Can you work these out from the model? Positions are in its coordinate system, mm. A direction names the side the tool comes from. Round coordinates to 2 decimals unless told otherwise and drop trailing zeros. Loops run counter-clockwise (first coordinate to the right, second up) from the corner with the lowest first, then second, coordinate; pieces in that order, holes last.
```python
from build123d import *

# Parameters (mm, degrees)
F1_DEPTH      = 6.4897
F1_DEPTH_BACK = 6.4897
F2_W          = 85.5599
F2_H          = 54.0004
F3_DEPTH      = 5.7277
F3_DEPTH_BACK = 5.7277
F4_R          = 0.762


with BuildPart() as f1:
    # F0 (on Top) → F1 (new body, two sides)
    with BuildSketch(Plane.XY) as f1_sk:
        Polygon((9.525, -27.7622), (9.525, 27.7622), (-9.525, 27.7622), (-9.525, 9.525), (-43.54195, 9.525), (-43.54195, -9.525), (-9.525, -9.525), (-9.525, -27.7622), align=None)
    extrude(amount=F1_DEPTH)
    extrude(f1_sk.sketch, amount=-F1_DEPTH_BACK)

    # F2 (on Top) → F3 (cut, two sides)
    with BuildSketch(Plane.XY) as f3_sk:
        Rectangle(F2_W, F2_H)
    extrude(amount=-F3_DEPTH, mode=Mode.SUBTRACT)
    extrude(f3_sk.sketch, amount=F3_DEPTH_BACK, mode=Mode.SUBTRACT)

    # F4
    f4_edges = [f1.edges().sort_by_distance(p)[0] for p in [
        (0, -27.7622, 6.4897),
        (0, -27.7622, -6.4897),
        (0, 27.7622, 6.4897),
        (0, 27.7622, -6.4897),
        (-43.54195, 0, -6.4897),
        (-43.54195, 0, 6.4897),
    ]]
    fillet(f4_edges, radius=F4_R)


solid = f1.part
```
(1) Which directions (+Z, -Z, +X, -X, +Y, -Y) give clear straight access to the entire face, cutting with the end or side of a thin tool? Please do faces 1 (the flat face through (-29, 9.525, -6)), 2 (the flat face through (-9.525, -20, -6)), 3 (the flat face through (0, 27, 0)), 4 (the flat face through (-11, 0, -5.728)), 5 (the flat face through (-42.78, 0, 0)).
(2) We'd pull the mould along Y, two halves only. Please class faces 6 (the flat face through (-9.525, 20, -6)), 7 (the flat face through (0, -27, 0)), 8 (the flat face through (0, -27.762, 0)): released by +Y, released by -Y, zero draft, split by the parting line, or undercut.
(3) Suppose I cut it at B-B (x = -18). Write out the boundary of the cut face in (y, z) (3 decimals), then the cut area to 3 significant figures.
(4) Suppose I cut it at D-D (x = 5.5). Write out the boundary of the cut face in (y, z).
(5) If I drill on line 1 (Z direction, x = -14.5, y = -3.5); line 2 (Y direction, x = 5, z = -3.5); line 3 (X direction, y = 2, z = -5.25), over which ranges is the centre line in solid material (lowest first)?
(6) Suppose I cut it at A-A (z = -2). Write out the boundary of the cut face in (x, y) (3 decimals).
Check result:
1. face 1: +Z, -Z, -X, +Y
1. face 2: +Z, -Z, -X, -Y
1. face 3: +X, -X
1. face 4: +X
1. face 5: +X, +Y, -Y
2. face 6: zero draft
2. face 7: undercut
2. face 8: released by -Y
3. outline: (-9.525, -6.49) - (9.525, -6.49) - (9.525, -5.728) - (-9.525, -5.728) - close; (-9.525, 5.728) - (9.525, 5.728) - (9.525, 6.49) - (-9.525, 6.49) - close
3. area: 29.0 mm2
4. outline: (-27.76, -5.73) arc R0.76 ccw to (-27, -6.49) - (27, -6.49) arc R0.76 ccw to (27.76, -5.73) - (27.76, 5.73) arc R0.76 ccw to (27, 6.49) - (-27, 6.49) arc R0.76 ccw to (-27.76, 5.73) - close; hole (-27, -5.73) - (27, -5.73) - (27, 5.73) - (-27, 5.73) - close
5. line 1: z = -6.49 to -5.73, 5.73 to 6.49
5. line 2: y = -27.76 to -27, 27 to 27.76
5. line 3: x = -43.54 to -42.78
6. outline: (-43.542, -9.525) - (-42.78, -9.525) - (-42.78, 9.525) - (-43.542, 9.525) - close; (-9.525, -27.762) - (9.525, -27.762) - (9.525, -27) - (-9.525, -27) - close; (-9.525, 27) - (9.525, 27) - (9.525, 27.762) - (-9.525, 27.762) - close
